Work out the finished part from the listing and answer in its coordinate system (mm). Round coordinates to 2 decimals unless told otherwise and drop trailing zeros. Write each loop counter-clockwise with the first axis right and the second up, starting at its lowest first coordinate (ties: lowest second). Pieces come first, ordered by that corner, then holes. Notation, with made-up numbers: (67, 31.5) -> (96, 31.5) arc R37 cw to (96, 67.5) -> close; hole circle Ø3 at (-32, -0.75). An arc over 180 degrees is marked (long way). One line per item, written item: value.
Autodesk Inventor part; units mm, degrees
ref_plane "Start plane" through (0, 0, 0) normal (0, 0, 1) x (1, 0, 0)
ref_plane "End plane" through (0, 0, 1080) normal (0, 0, 1) x (1, 0, 0)
ref_plane "Work Plane4" through (0, 10, 1080) normal (0, 0, 1) x (1, 0, 0)
ref_plane "Start plane" through (0, 0, 0) normal (0, 0, 1) x (1, 0, 0)
ref_plane "End plane" through (0, 0, 1080) normal (0, 0, 1) x (1, 0, 0)
sketch "Sketch" plane through (0, 0, 0) normal (0, 0, 1) x (1, 0, 0)
  line L0 (-10, -6) -> (-10, 6)
  line L1 (-6, 10) -> (6, 10)
  line L2 (10, 6) -> (10, -6)
  line L3 (6, -10) -> (-6, -10)
  arc A0 (-10, -6) -> (-6, -10) centre (-6, -6) ccw
  arc A1 (10, 6) -> (6, 10) centre (6, 6) ccw
  arc A2 (-6, 10) -> (-10, 6) centre (-6, 6) ccw
  arc A3 (6, -10) -> (10, -6) centre (6, -6) ccw
  arc A4 (-6, 8) -> (-8, 6) centre (-6, 6) ccw
  line L4 (-6, 8) -> (6, 8)
  arc A5 (8, 6) -> (6, 8) centre (6, 6) ccw
  line L5 (8, 6) -> (8, -6)
  arc A6 (6, -8) -> (8, -6) centre (6, -6) ccw
  line L6 (6, -8) -> (-6, -8)
  arc A7 (-8, -6) -> (-6, -8) centre (-6, -6) ccw
  line L7 (-8, -6) -> (-8, 6)
  line L8 (0, 15.1598) -> (0, -15.1598) construction
  line L9 (-15.1598, 0) -> (15.1598, 0) construction
  dimension "d7" = 4
  dimension "d9" = 20
  dimension "d11" = 20
  dimension "d12" = 2
  dimension "d15" = 10
  dimension "d16" = 10
extrude "Body" add sketch "Sketch" along normal up to surface (1080 mm away) from surface at 0
sketch "Sketch3" plane through (0, 0, 0) normal (0, 0, 1) x (1, 0, 0)
  line L0 (0, 0) -> (10, 0)
ref_plane "Work Plane3" through (0, 0, 0) normal (0, -1, 0) x (1, 0, 0)
sketch "Sketch4" plane through (0, 0, 0) normal (0, -1, 0) x (1, 0, 0)
  line L0 (-2, 0) -> (12, 0)
  line L1 (-2, 1080) -> (12, 1080)
  dimension "d18" = 1080
ref_plane "Work Plane4" through (0, 10, 1080) normal (0, 0, 1) x (1, 0, 0)
split "Split1" plane through (0, 10, 1080) removes the side toward (0, 0, 1)
equation "\"d7\" = G_IR"
equation "\"d9\" = G_W"
equation "\"d11\" = G_H"
equation "\"d12\" = G_T"
equation "\"d15\" = 0.5 * d9"
equation "\"d16\" = 0.5 * d11"
equation "\"d3\" = G_L"
equation "\"G_W\" = 20"
equation "\"G_H\" = 20"
equation "\"G_T\" = 2"
equation "\"G_IR\" = 4"
equation "\"G_L\" = d18"
equation "\"G_OFFSET_START\" = 0"
properties part number "ISO 4019 - 20x20x2 - 1080" material "Steel, Mild"
(1) Consider probe 1 along Y at (x, z) = (-4.25, 243); probe 2 along Y at (x, z) = (6.5, 402.5). Determine where each line is inside the solid, lowest interval first.
Reported:
probe 1: y = -10 to -8, 8 to 10
probe 2: y = -9.97 to -7.94, 7.94 to 9.97
(2) Find section A-A on x = 1.75. Give the vertices of the cut face in (y, z).
Reported:
outline: (-10, 0) -> (-8, 0) -> (-8, 1080) -> (-10, 1080) -> close; (8, 0) -> (10, 0) -> (10, 1080) -> (8, 1080) -> close
(3) Find section C-C on z = 319. Give the vertices of the cut face in (x, y).
Reported:
outline: (-10, -6) arc R4 ccw to (-6, -10) -> (6, -10) arc R4 ccw to (10, -6) -> (10, 6) arc R4 ccw to (6, 10) -> (-6, 10) arc R4 ccw to (-10, 6) -> close; hole (-8, -6) arc R2 ccw to (-6, -8) -> (6, -8) arc R2 ccw to (8, -6) -> (8, 6) arc R2 ccw to (6, 8) -> (-6, 8) arc R2 ccw to (-8, 6) -> close
